```python
from build123d import *

# Parameters (mm, degrees)
SKETCH1_R           = 12
SKETCH1_R_2         = 1.5
SKETCH1_R_3         = 2
BOSS_EXTRUDE1_DEPTH = 7
BOSS_EXTRUDE2_DEPTH = 6
BOSS_EXTRUDE3_START = -99
BOSS_EXTRUDE3_DEPTH = 6
BOSS_EXTRUDE4_START = -54
BOSS_EXTRUDE4_DEPTH = 6
SKETCH3_W           = 12
SKETCH3_H           = 37
SKETCH3_R           = 2
BOSS_EXTRUDE5_DEPTH = 6
SKETCH4_W           = 12
SKETCH4_H           = 18.5
CUT_EXTRUDE1_DEPTH  = 10
CHAMFER1_SIZE       = 2
CHAMFER2_SIZE       = 2


with BuildPart() as part:
    # Sketch1 → Boss-Extrude1 (new body)
    with BuildSketch(Plane.XY):
        Polygon((0, 0), (45, 0), (45, 27), (93, 27), (93, 0), (99, 0), (99, 38), (0, 38), align=None)
        with Locations((17.5, 19)):
            Circle(SKETCH1_R, mode=Mode.SUBTRACT)
        with Locations((5, 29)):
            Circle(SKETCH1_R_2, mode=Mode.SUBTRACT)
        with Locations((5, 9)):
            Circle(SKETCH1_R_2, mode=Mode.SUBTRACT)
        with Locations((30, 9)):
            Circle(SKETCH1_R_2, mode=Mode.SUBTRACT)
        with Locations((30, 29)):
            Circle(SKETCH1_R_2, mode=Mode.SUBTRACT)
        with Locations((69, 33)):
            Circle(SKETCH1_R_3, mode=Mode.SUBTRACT)
    extrude(amount=BOSS_EXTRUDE1_DEPTH)

    # Sketch2 → Boss-Extrude2 (add)
    with BuildSketch(Plane(origin=(99, 0, 0), x_dir=(0, 0, -1), z_dir=(1, 0, 0))):
        Polygon((-37, 0), (-7, 0), (0, 0), (0, 38), (-7, 38), (-37, 6), align=None)
    extrude(amount=-BOSS_EXTRUDE2_DEPTH)

    # Sketch2<3> → Boss-Extrude3 (add)
    with BuildSketch(Plane(origin=(99, 0, 0), x_dir=(0, 0, -1), z_dir=(1, 0, 0)).offset(BOSS_EXTRUDE3_START)):
        Polygon((-37, 0), (-7, 0), (0, 0), (0, 38), (-7, 38), (-37, 6), align=None)
    extrude(amount=-BOSS_EXTRUDE3_DEPTH)

    # Sketch2<4> → Boss-Extrude4 (add)
    with BuildSketch(Plane(origin=(99, 0, 0), x_dir=(0, 0, -1), z_dir=(1, 0, 0)).offset(BOSS_EXTRUDE4_START)):
        Polygon((-37, 0), (-7, 0), (0, 0), (0, 38), (-7, 38), (-37, 6), align=None)
    extrude(amount=-BOSS_EXTRUDE4_DEPTH)

    # Sketch3 → Boss-Extrude5 (add)
    # profile 1 of 2: a face of its own
    with BuildSketch(Plane(origin=(0, 0, 0), x_dir=(-1, 0, 0), z_dir=(0, -1, 0))):
        with Locations((12, -18.5)):
            Rectangle(SKETCH3_W, SKETCH3_H)
        with Locations(Location((12, -31, 0), (0, 0, 90))):
            Circle(SKETCH3_R, mode=Mode.SUBTRACT)
        with Locations(Location((12, -6, 0), (0, 0, 90))):
            Circle(SKETCH3_R, mode=Mode.SUBTRACT)
    # profile 2 of 2: a face of its own
    with BuildSketch(Plane(origin=(0, 0, 0), x_dir=(-1, 0, 0), z_dir=(0, -1, 0))):
        with Locations((-105, -18.5)):
            Rectangle(SKETCH3_W, SKETCH3_H)
        with Locations(Location((-105, -31, 0), (0, 0, 270))):
            Circle(SKETCH3_R, mode=Mode.SUBTRACT)
        with Locations(Location((-105, -6, 0), (0, 0, 270))):
            Circle(SKETCH3_R, mode=Mode.SUBTRACT)
    extrude(amount=-BOSS_EXTRUDE5_DEPTH)

    # Sketch4 → Cut-Extrude1 (cut)
    with BuildSketch(Plane(origin=(0, 6, 0), x_dir=(1, 0, 0), z_dir=(0, 1, 0))):
        with Locations((-12, -9.25)):
            Rectangle(SKETCH4_W, SKETCH4_H)
    extrude(amount=-CUT_EXTRUDE1_DEPTH, mode=Mode.SUBTRACT)

    # Chamfer1
    chamfer1_edges = [part.edges().sort_by_distance(p)[0] for p in [
        (5.5, 19, 0),
        (69, 38, 7),
        (19.5, 38, 7),
        (111, 0, 18.5),
        (111, 6, 18.5),
        (19.5, 0, 7),
        (0, 0, 22),
        (93, 0, 18.5),
        (93, 3, 37),
        (102, 0, 37),
        (0, 3, 37),
        (39, 0, 22),
        (42, 0, 37),
        (45, 0, 18.5),
        (-9, 0, 37),
        (-18, 3, 37),
        (-18, 0, 27.75),
        (-18, 6, 27.75),
        (19.5, 0, 0),
        (45, 13.5, 0),
        (69, 27, 0),
        (93, 13.5, 0),
        (102, 0, 0),
        (111, 3, 37),
        (111, 3, 0),
        (105, 6, 0),
        (99, 22, 22),
        (99, 38, 3.5),
        (-6, 22, 22),
        (-6, 38, 3.5),
        (-6, 19, 0),
        (99, 22, 0),
        (46.5, 38, 0),
        (-12, 0, 18.5),
        (-12, 6, 18.5),
        (-6, 0, 9.25),
    ]]
    chamfer(chamfer1_edges, length=CHAMFER1_SIZE)

    # Chamfer2
    # the kernel refuses this chamfer: 2 mm, written as the material it takes off along each edge
    with BuildSketch(Plane(origin=(97, 6, 37), x_dir=(0, 0.027495876610588235, -0.9996219169112968), z_dir=(1, 0, 0))) as chamfer2_piece_1_section:
        Polygon((CHAMFER2_SIZE * 0.999621916911, -CHAMFER2_SIZE * 0.0274958766106), (-CHAMFER2_SIZE * 0.0274958766106, -CHAMFER2_SIZE * 0.999621916911), (0, 0), align=None)
    chamfer2_piece_1 = extrude(amount=17.143365976, mode=Mode.PRIVATE)
    chamfer2_piece_1 = split(chamfer2_piece_1, bisect_by=Plane(origin=(100.7856843, 3.388099041, 34.25949849), z_dir=(0.7071067811865475, 0.4836194101643707, 0.5158607041753291)), keep=Keep.TOP, mode=Mode.PRIVATE)
    add(chamfer2_piece_1, mode=Mode.SUBTRACT)
    with BuildSketch(Plane(origin=(-4, 6, 37), x_dir=(-1.1675093231223383e-15, 0.027495876610589956, -0.9996219169112965), z_dir=(-1, 0, 0))) as chamfer2_piece_2_section:
        Polygon((CHAMFER2_SIZE * 0.999621916911, CHAMFER2_SIZE * 0.0274958766106), (-CHAMFER2_SIZE * 0.0274958766106, CHAMFER2_SIZE * 0.999621916911), (0, 0), align=None)
    chamfer2_piece_2 = extrude(amount=17.143365976, mode=Mode.PRIVATE)
    chamfer2_piece_2 = split(chamfer2_piece_2, bisect_by=Plane(origin=(-7.7856843, 3.388099041, 34.25949849), z_dir=(-0.7071067811865475, 0.4836194101643707, 0.5158607041753291)), keep=Keep.TOP, mode=Mode.PRIVATE)
    add(chamfer2_piece_2, mode=Mode.SUBTRACT)
    with BuildSketch(Plane(origin=(0, 41.752276834, 3.482240468), x_dir=(0.027495876610586428, -0.6836825423068311, -0.72926137846062), z_dir=(0, -0.7295372041400852, 0.6839411288813297))) as chamfer2_piece_3_section:
        Polygon((CHAMFER2_SIZE * 0.999621916911, -CHAMFER2_SIZE * 0.0274958766106), (-CHAMFER2_SIZE * 0.0274958766106, -CHAMFER2_SIZE * 0.999621916911), (0, 0), align=None)
    chamfer2_piece_3 = extrude(amount=51.225928058, mode=Mode.PRIVATE)
    chamfer2_piece_3 = split(chamfer2_piece_3, bisect_by=Plane(origin=(-0.581475565, 36.992815088, 6.007184912), z_dir=(0, 0.7071067811865476, 0.7071067811865476)), keep=Keep.TOP, mode=Mode.PRIVATE)
    add(chamfer2_piece_3, mode=Mode.SUBTRACT)
    with BuildSketch(Plane(origin=(0, 41.752276834, 3.482240468), x_dir=(0.027495876610586428, -0.6836825423068311, -0.72926137846062), z_dir=(0, -0.7295372041400852, 0.6839411288813297))) as chamfer2_piece_4_section:
        Polygon((CHAMFER2_SIZE * 0.999621916911, -CHAMFER2_SIZE * 0.0274958766106), (-CHAMFER2_SIZE * 0.0274958766106, -CHAMFER2_SIZE * 0.999621916911), (0, 0), align=None)
    chamfer2_piece_4 = extrude(amount=51.225928058, mode=Mode.PRIVATE)
    chamfer2_piece_4 = split(chamfer2_piece_4, bisect_by=Plane(origin=(-0.512278585, 16.479410692, 7), z_dir=(0, 0, 1)), keep=Keep.TOP, mode=Mode.PRIVATE)
    add(chamfer2_piece_4, mode=Mode.SUBTRACT)
    with BuildSketch(Plane(origin=(93, 41.752276834, 3.482240468), x_dir=(-0.027495876610589116, -0.683682542306831, -0.7292613784606198), z_dir=(0, -0.7295372041400852, 0.6839411288813297))) as chamfer2_piece_5_section:
        Polygon((CHAMFER2_SIZE * 0.999621916911, CHAMFER2_SIZE * 0.0274958766106), (-CHAMFER2_SIZE * 0.0274958766106, CHAMFER2_SIZE * 0.999621916911), (0, 0), align=None)
    chamfer2_piece_5 = extrude(amount=51.225928058, mode=Mode.PRIVATE)
    chamfer2_piece_5 = split(chamfer2_piece_5, bisect_by=Plane(origin=(93.581475565, 36.992815088, 6.007184912), z_dir=(0, 0.7071067811865476, 0.7071067811865476)), keep=Keep.TOP, mode=Mode.PRIVATE)
    add(chamfer2_piece_5, mode=Mode.SUBTRACT)
    with BuildSketch(Plane(origin=(93, 41.752276834, 3.482240468), x_dir=(-0.027495876610589116, -0.683682542306831, -0.7292613784606198), z_dir=(0, -0.7295372041400852, 0.6839411288813297))) as chamfer2_piece_6_section:
        Polygon((CHAMFER2_SIZE * 0.999621916911, CHAMFER2_SIZE * 0.0274958766106), (-CHAMFER2_SIZE * 0.0274958766106, CHAMFER2_SIZE * 0.999621916911), (0, 0), align=None)
    chamfer2_piece_6 = extrude(amount=51.225928058, mode=Mode.PRIVATE)
    chamfer2_piece_6 = split(chamfer2_piece_6, bisect_by=Plane(origin=(93.512278585, 16.479410692, 7), z_dir=(0, 0, 1)), keep=Keep.TOP, mode=Mode.PRIVATE)
    add(chamfer2_piece_6, mode=Mode.SUBTRACT)
    with BuildSketch(Plane(origin=(39, 41.752276834, 3.482240468), x_dir=(0.9996219169112968, 0.01880556088862619, 0.020059264947867937), z_dir=(0, -0.7295372041400852, 0.6839411288813297))) as chamfer2_piece_7_section:
        Polygon((CHAMFER2_SIZE * 0.999621916911, -CHAMFER2_SIZE * 0.0274958766106), (-CHAMFER2_SIZE * 0.0274958766106, -CHAMFER2_SIZE * 0.999621916911), (0, 0), align=None)
    chamfer2_piece_7 = extrude(amount=54.150156351, mode=Mode.PRIVATE)
    chamfer2_piece_7 = split(chamfer2_piece_7, bisect_by=Plane(origin=(39.581475565, 36.992815088, 6.007184912), z_dir=(0, 0.7071067811865476, 0.7071067811865476)), keep=Keep.TOP, mode=Mode.PRIVATE)
    add(chamfer2_piece_7, mode=Mode.SUBTRACT)
    with BuildSketch(Plane(origin=(39, 41.752276834, 3.482240468), x_dir=(0.9996219169112968, 0.01880556088862619, 0.020059264947867937), z_dir=(0, -0.7295372041400852, 0.6839411288813297))) as chamfer2_piece_8_section:
        Polygon((CHAMFER2_SIZE * 0.999621916911, -CHAMFER2_SIZE * 0.0274958766106), (-CHAMFER2_SIZE * 0.0274958766106, -CHAMFER2_SIZE * 0.999621916911), (0, 0), align=None)
    chamfer2_piece_8 = extrude(amount=54.150156351, mode=Mode.PRIVATE)
    chamfer2_piece_8 = split(chamfer2_piece_8, bisect_by=Plane(origin=(39.51114873, 15.48496609, 7), z_dir=(0, 0, 1)), keep=Keep.TOP, mode=Mode.PRIVATE)
    add(chamfer2_piece_8, mode=Mode.SUBTRACT)
    with BuildSketch(Plane(origin=(45, 41.752276834, 3.482240468), x_dir=(0.027495876610585664, -0.6836825423068311, -0.7292613784606199), z_dir=(0, -0.7295372041400852, 0.6839411288813297))) as chamfer2_piece_9_section:
        Polygon((CHAMFER2_SIZE * 0.999621916911, -CHAMFER2_SIZE * 0.0274958766106), (-CHAMFER2_SIZE * 0.0274958766106, -CHAMFER2_SIZE * 0.999621916911), (0, 0), align=None)
    chamfer2_piece_9 = extrude(amount=54.150156351, mode=Mode.PRIVATE)
    chamfer2_piece_9 = split(chamfer2_piece_9, bisect_by=Plane(origin=(44.418524435, 36.992815088, 6.007184912), z_dir=(0, 0.7071067811865476, 0.7071067811865476)), keep=Keep.TOP, mode=Mode.PRIVATE)
    add(chamfer2_piece_9, mode=Mode.SUBTRACT)
    with BuildSketch(Plane(origin=(45, 41.752276834, 3.482240468), x_dir=(0.027495876610585664, -0.6836825423068311, -0.7292613784606199), z_dir=(0, -0.7295372041400852, 0.6839411288813297))) as chamfer2_piece_10_section:
        Polygon((CHAMFER2_SIZE * 0.999621916911, -CHAMFER2_SIZE * 0.0274958766106), (-CHAMFER2_SIZE * 0.0274958766106, -CHAMFER2_SIZE * 0.999621916911), (0, 0), align=None)
    chamfer2_piece_10 = extrude(amount=54.150156351, mode=Mode.PRIVATE)
    chamfer2_piece_10 = split(chamfer2_piece_10, bisect_by=Plane(origin=(44.48885127, 15.48496609, 7), z_dir=(0, 0, 1)), keep=Keep.TOP, mode=Mode.PRIVATE)
    add(chamfer2_piece_10, mode=Mode.SUBTRACT)


solid = part.part
```
The listing builds one solid part. Answer for the finished solid, in the listing's coordinates (mm). A direction names the side the tool comes from. Give positions to 0.01 mm unless a question says otherwise; leave off trailing zeros. Write each loop counter-clockwise with the first axis right and the second up, starting at its lowest first coordinate (ties: lowest second). Pieces come first, ordered by that corner, then holes. Notation, with made-up numbers: M 25,80 L 42,80 A13 ccw 42,96 Z; hole C 31.25,74.5 d3. An arc over 180 degrees is marked long. Write each question's results on one line, items separated by ' | '.
Q1. Section A-A, the plane x = 17.5 is taken. Write down the section's boundary in (y, z).
Output values:
outline: M 0,2 L 2,0 L 5,0 L 7,2 L 7,7 L 2,7 L 0,5 Z; M 31,2 L 33,0 L 36,0 L 38,2 L 38,5 L 36,7 L 31,7 Z
Q2. Consider L1, parallel to Z at x = 105, y = 3; L2, parallel to X at y = 2.9, z = 6; L3, parallel to X at y = 4.6, z = 31. Determine where each line is inside the solid, lowest interval first. Write a range as from..to.
Output values:
L1: 0..4, 8..29, 33..37 | L2: -6..45, 93..103, 107..111 | L3: -17.4..-14, -10..0, 39..45, 93..103, 107..110.4
Q3. Section B-B, the plane x = 105 is taken. Write down the section's boundary in (y, z), then the cut area to 3 significant figures.
Output values:
outline: M 0,2 L 2,0 L 4,0 L 6,2 L 6,4 L 0,4 Z; M 0,8 L 6,8 L 6,29 L 0,29 Z; M 0,33 L 6,33 L 6,35 L 4,37 L 2,37 L 0,35 Z | area: 166 mm2
Q4. Section C-C, the plane z = 25 is taken. Count the separate pieces of the cut face and the enclosed holes in it, then the cut area to 3 significant figures.
Output values:
separate pieces: 3 | enclosed holes: 0 | area: 449 mm2
Q5. For a pull along X with two mould halves and no side action, classify faces 5 (the cylindrical face through (5.69, 7.67, 3.45)), 6 (the flat face through (104, 6, 18)), 7 (the flat face through (99, 18, 15)) as released by +X, released by -X, zero draft, split by the parting line, or undercut.
Output values:
face 5: undercut | face 6: zero draft | face 7: released by +X
Q6. Flat-ended cylindrical pins translate along their axes: P1, Ø15, axis at y = 17, z = 21, coming from the +X side; P2, Ø5, axis at x = 105, z = 31, coming from the +Y side; P3, Ø2, axis at y = 12, z = 31, coming from the +X side; P4, Ø6, axis at x = 31, y = 18, coming from the -Z side. Find the tip coordinate at first contact, or state that the pin passes through.
Output values:
P1: x = 99 | P2: y = 6 | P3: x = 98.27 | P4: z = 0
Q7. Section D-D, the plane x = 35 is taken. Write down the section's boundary in (y, z), then the cut area to 3 significant figures.
Output values:
outline: M 0,2 L 2,0 L 36,0 L 38,2 L 38,5 L 36,7 L 2,7 L 0,5 Z | area: 258 mm2
Q8. A tool of negligible diameter and unlimited length cuts with its end or side. For faces 1 (the flat face through (11, 0, 4)), 2 (the flat face through (0, 15, 18)), 3 (the flat face through (69, 27, 4)), 4 (the flat face through (44.01, 21.27, 21.3)), from which of +Z, -Z, +X, -X, +Y, -Y can it reach the whole face along a straight path? Write none if from no direction.
Output values:
face 1: +Z, -Z, +X, -X, -Y | face 2: +Z, +Y, -Y | face 3: +Z, -Z, -Y | face 4: +Z, +Y
